Print and shaded views of the part. All mm, measured from the part's lowest x, y and z. A direction names the side the tool comes from. Round coordinates to 2 decimals unless told otherwise and drop trailing zeros. Loops run counter-clockwise (first coordinate to the right, second up) from the corner with the lowest first, then second, coordinate; pieces in that order, holes last. Notation, with made-up numbers: (20, -20.5) -> (76, -20.5) arc R18 ccw to (76, -3.5) -> close; hole circle Ø7 at (16, -35). An arc over 180 degrees is marked (long way). Answer as CSV lines item,"result".
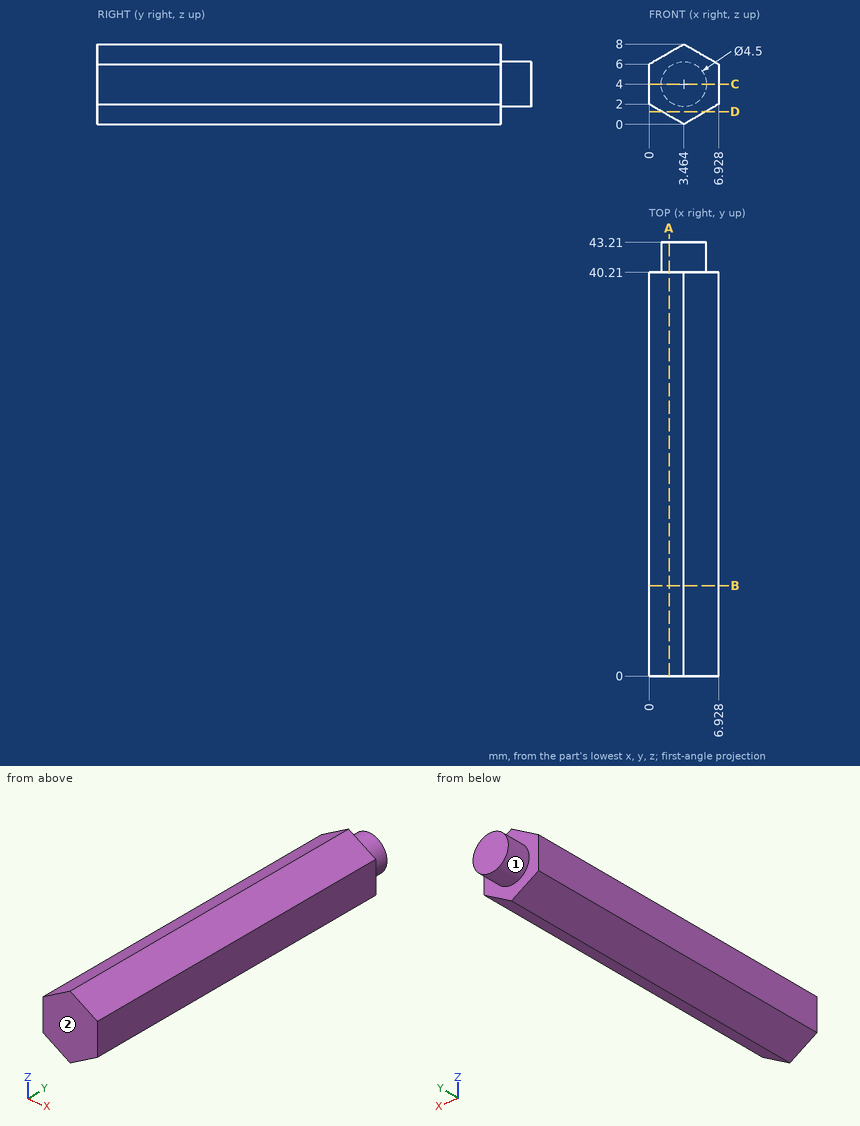
Q1. Slice it at C-C, the plane z = 4. Give the cut face in (x, y).
Results:
outline,"(0, 0) -> (6.93, 0) -> (6.93, 40.21) -> (5.71, 40.21) -> (5.71, 43.21) -> (1.21, 43.21) -> (1.21, 40.21) -> (0, 40.21) -> close"
Q2. Slice it at A-A, the plane x = 2. Give the cut face in (y, z) (1 decimal), and give its area (3 significant figures).
Results:
outline,"(0, 0.8) -> (40.2, 0.8) -> (40.2, 2.3) -> (43.2, 2.3) -> (43.2, 5.7) -> (40.2, 5.7) -> (40.2, 7.2) -> (0, 7.2) -> close"
area,"264 mm2"
Q3. Tool access for the marked faces 1 and 2: list every direction of +Z, -Z, +X, -X, +Y, -Y with a clear straight run to the whole face (end or side of a thin tool).
Results:
face 1,"+Y"
face 2,"+Z, -Z, +X, -X, -Y"
Q4. Drop a flat-ended pin along its axis: pin 1 Ø3 at (x, z) = (2.5, 3.5) entering from -Y. Give the stop position or say it passes through.
Results:
pin 1,"y = 0"
Q5. Slice it at B-B, the plane y = 9. Give the cut face in (x, z), and give its area (3 significant figures).
Results:
outline,"(0, 2) -> (3.46, 0) -> (6.93, 2) -> (6.93, 6) -> (3.46, 8) -> (0, 6) -> close"
area,"41.6 mm2"
Q6. Slice it at D-D, the plane z = 1.25. Give the cut face in (x, y), and give its area (3 significant figures).
Results:
outline,"(1.3, 0) -> (5.63, 0) -> (5.63, 40.21) -> (1.3, 40.21) -> close"
area,"174 mm2"
Q7. Probe L1, parallel to Y at x = 3.25, z = 1; L2, parallel to Z at x = 6, y = 18.5; L3, parallel to Z at x = 2, y = 10 (1 decimal). List the from-to ranges inside material, lowest first. Write a range as [from, to].
Results:
L1,"[0, 40.21]"
L2,"[1.46, 6.54]"
L3,"[0.8, 7.2]"
